Can you work these out from the model? Positions are in its coordinate system, mm. A direction names the side the tool comes from. Round coordinates to 2 decimals unless told otherwise and drop trailing zeros. Write each loop counter-clockwise with the first axis right and the second up, starting at its lowest first coordinate (ties: lowest second). Pieces come first, ordered by that corner, then holes. Notation, with made-up numbers: (-36.75, 55) - (-14.75, 55) arc R14 cw to (-14.75, 72) - close; hole circle Ø7 at (84.5, -7). An arc over 180 degrees is marked (long way). One line per item, written item: value. Start each with the question number.
(1) I want a section at A-A on z = 4.75. List the corners of the cut face in (x, y) for me, plus the area to 3 significant figures.
(2) On a 3-axis mill with a long thin cutter (end or side, diameter ignored), from which of +Z, -Z, +X, -X, +Y, -Y can I reach the whole of each face in a straight line? I mean faces 1 (the face through (4.7, 3, -11)), 2 (the face through (-6.6, 1.46, -2.8)), 3 (the face through (4.7, 4, 10)), 4 (the face through (-1, 3, -10)), 5 (the face through (-6.4, 3.2, -1.85)). Say none if no direction works.
(3) I want a section at C-C on z = -4.75. List the corners of the cut face in (x, y) for me.
(4) I want a section at B-B on x = 2.2. List the corners of the cut face in (y, z) for me.
(5) If I drill on L1, parallel to Z at x = 2.2, y = 4.25; L2, parallel to X at y = 1.75, z = 4.75; L3, parallel to X at y = 1.75, z = -4.75, over which ranges is the centre line in solid material (lowest first)? Write a range as from..to.
(6) I'm going to push flat-ended pins straight in: pin 1 Ø3 at (y, z) = (4.5, 2.5) entering from -X; pin 2 Ø1 at (x, y) = (-0.5, 1.5) entering from -Z; pin 3 Ø1.5 at (y, z) = (3, -11) entering from -X. Where does each tip first touch, or does it pass through?
(7) Thinking about a two-plate mould opening in Z: for faces 6 (the face through (4.928, 3.4, 9.667)), 7 (the face through (-5, 3, 5)), 8 (the face through (1.93, 3.22, -3.53)), 9 (the face through (0, 3, 10)), which applies, +Z half, -Z half, draft (parallel to the pull), parting line (faces both ways), or undercut?
(8) I want a section at D-D on x = -0.5. List the corners of the cut face in (y, z) for me, plus the area to 3 significant figures.
Autodesk Inventor part; units mm, degrees
ref_plane "YZ Plane" through (0, 0, 0) normal (1, 0, 0) x (0, 1, 0)
ref_plane "XZ Plane" through (0, 0, 0) normal (0, 1, 0) x (-1, 0, 0)
ref_plane "XY Plane" through (0, 0, 0) normal (0, 0, 1) x (1, 0, 0)
sketch "Skizze1" plane through (0, 0, 0) normal (0, 1, 0) x (-1, 0, 0)
  line L0 (5, 10) -> (-5, 10)
  line L1 (-5, 10) -> (-5, -10)
  line L2 (-5, -10) -> (5, -10)
  line L3 (5, -10) -> (5, 10)
  line L4 (5, 10) -> (-5, -10) construction
  line L5 (-5, 10) -> (5, -10) construction
  line L6 (5, -10) -> (6, -10)
  line L7 (6, -10) -> (6, 0)
  line L8 (6, 0) -> (5, 0)
  line L9 (5, 0) -> (5, -10)
  point P0 (0, 0)
  dimension "d0" = 10
  dimension "d1" = 20
  dimension "d2" = 1
extrude "Extrusion1" add sketch "Skizze1" along normal blind 6.35
sketch "Skizze2" plane through (-6, 0, -10) normal (-1, 0, 0) x (0, 0, 1)
  line L0 (0, 0) -> (0, 6.35)
  line L1 (0, 0) -> (10, 0)
  line L2 (0, 6.35) -> (8.15, 6.35)
  line L3 (8.15, 6.35) -> (8.15, 0)
  line L4 (8.15, 0) -> (0, 0)
  line L5 (0, 0) -> (0, 6.35)
  line L6 (8.15, 6.35) -> (6.15, 6.35)
  line L7 (6.15, 6.35) -> (6.15, 0)
  line L8 (6.15, 0) -> (8.15, 0)
  line L9 (8.15, 0) -> (8.15, 6.35)
  line L10 (6.15, 4.89) -> (8.15, 4.89)
  line L11 (8.15, 4.89) -> (8.15, 1.46)
  line L12 (8.15, 1.46) -> (6.15, 1.46)
  line L13 (6.15, 1.46) -> (6.15, 4.89)
  line L14 (6.15, 4.89) -> (8.15, 1.46) construction
  line L15 (8.15, 4.89) -> (6.15, 1.46) construction
  point P0 (7.15, 3.175)
  point P1 (8.15, 1.46)
  dimension "d5" = 8.15
  dimension "d6" = 2
  dimension "d7" = 2
  dimension "d8" = 3.43
extrude "Extrusion2" add sketch "Skizze2" along normal blind 1.15 contours L7 L10 L3 L12
sketch "Skizze3" plane through (-6, 4.89, -1.85) normal (0, 1, 0) x (1, 0, 0)
  line L0 (0, 2) -> (0, 0)
  line L1 (0, 2) -> (-1.15, 2)
  line L2 (-1.15, 0) -> (-1.15, 2)
  line L3 (0, 0) -> (-1.15, 0)
  circle A0 centre (1.35, 1) radius 2.5
  point P0 (6, -1.85)
  point P1 (-1.15, 1)
  point P2 (-0.9413, 0)
  point P3 (-0.9413, 2)
  dimension "d11" = 5
extrude "Extrusion3" cut sketch "Skizze3" against normal through all contours A0 L2 L1 | L3 L2 A0
fillet "Rundung1" radius 0.2 2 edges at (-6.9413, 3.175, -1.85) (-6.9413, 3.175, -3.85)
chamfer "Fase1" distance 1 angle 45 1 edges at (-6, 3.175, 0)
fillet "Rundung2" radius 0.2 4 edges at (-5, 3.175, 10) (5, 3.175, 10) (5, 3.175, -10) (-6, 3.175, -10)
move faces "Verschieben1" translate (-0.4, 0, 0) faces at (4.8149, 2.1167, 9.9994) (4.936, 2.1167, -9.9466) (5, 2.1167, 3.2667)
sketch "Skizze4" plane through (4.6, 0, 9.8) normal (1, 0, 0) x (0, 0, -1)
  line L0 (19.6, 6.35) -> (19.6, 0)
  line L1 (0, 6.35) -> (19.6, 6.35)
  line L2 (0, 0) -> (0, 6.35)
  line L3 (0, 0) -> (19.6, 0)
  line L4 (1.95, 4.725) -> (17.65, 4.725)
  line L5 (17.65, 4.725) -> (17.65, 1.625)
  line L6 (17.65, 1.625) -> (1.95, 1.625)
  line L7 (1.95, 1.625) -> (1.95, 4.725)
  line L8 (9.8, 0) -> (9.8, 6.35)
  line L9 (1.95, 4.725) -> (17.65, 1.625) construction
  line L10 (17.65, 4.725) -> (1.95, 1.625) construction
  line L11 (1.5, 4.725) -> (18.1, 4.725)
  line L12 (18.1, 4.725) -> (18.1, 1.625)
  line L13 (18.1, 1.625) -> (1.5, 1.625)
  line L14 (1.5, 1.625) -> (1.5, 4.725)
  line L15 (1.5, 4.725) -> (18.1, 1.625) construction
  line L16 (18.1, 4.725) -> (1.5, 1.625) construction
  line L17 (9.8, 4.725) -> (9.35, 4.725)
  line L18 (9.35, 4.725) -> (9.35, 1.625)
  line L19 (9.35, 1.625) -> (9.8, 1.625)
  line L20 (9.8, 1.625) -> (9.8, 4.725)
  point P0 (9.8, 3.175)
  point P1 (9.8, 3.175)
  point P2 (17.65, 4.725)
  point P3 (17.65, 1.625)
  point P4 (9.35, 4.725)
  point P5 (9.8, 1.625)
  point P6 (9.8, 4.725)
  point P7 (1.95, 1.625)
  point P8 (1.95, 4.725)
  dimension "d22" = 15.7
  dimension "d23" = 3.1
  dimension "d24" = 16.6
  dimension "d25" = 0.45
extrude "Extrusion4" add sketch "Skizze4" along normal blind 0.55 contours L8 L6 L18 L4 | L11 L12 L13 L5 | L7 L13 L14 L11
sketch "Skizze5" plane through (4.6, 4.725, 8.3) normal (0, 1, 0) x (1, 0, 0)
  line L0 (0, 0) -> (0, 0.45)
  line L1 (0, 0) -> (0.55, 0)
  line L2 (0.55, 0.45) -> (0.55, 0)
  line L3 (0, 0.45) -> (0.55, 0.45)
  line L4 (0, 16.15) -> (0, 16.6)
  line L5 (0, 16.15) -> (0.55, 16.15)
  line L6 (0.55, 16.6) -> (0.55, 16.15)
  line L7 (0, 16.6) -> (0.55, 16.6)
  line L8 (1, -4.015) -> (0.1, -4.015)
  line L9 (0.1, -4.015) -> (0.1, 20.615)
  line L10 (0.1, 20.615) -> (1, 20.615)
  line L11 (1, 20.615) -> (1, -4.015)
  line L12 (0.55, 7.85) -> (0.55, 8.3)
  line L13 (1, -4.015) -> (0.1, 20.615) construction
  line L14 (0.1, -4.015) -> (1, 20.615) construction
  line L15 (0.55, 20.615) -> (0.55, -4.015)
  point P0 (-4.6, 8.3)
  point P1 (0.1, 16.6)
  point P2 (0.1, 0)
  dimension "d28" = 0.9
  dimension "d29" = 24.63
extrude "Extrusion5" add sketch "Skizze5" against normal up to surface (3.1 mm away) contours L1 L15 L8 L9 | L9 L10 L15 L7
fillet "Rundung3" radius 0.2 2 edges at (5.15, 3.175, -7.85) (5.15, 3.175, 7.85)
fillet "Rundung4" radius 0.1 2 edges at (4.7, 3.175, -8.3) (4.7, 3.175, 8.3)
fillet "Rundung5" radius 0.1 2 edges at (5.15, 3.175, 0.45) (5.15, 3.175, 0)
sketch "Skizze6" plane through (5.15, 0, 9.8) normal (1, 0, 0) x (0, 0, -1)
  line L0 (1.75, 4.725) -> (1.75, 1.625)
  line L1 (1.75, 4.725) -> (-2.515, 4.725)
  line L2 (-2.515, 4.725) -> (-2.515, 1.625)
  line L3 (-2.515, 1.625) -> (1.75, 1.625)
  line L4 (17.85, 1.625) -> (17.85, 4.725)
  line L5 (17.85, 1.625) -> (22.115, 1.625)
  line L6 (22.115, 4.725) -> (22.115, 1.625)
  line L7 (17.85, 4.725) -> (22.115, 4.725)
  circle A0 centre (-0.5825, 3.175) radius 0.75
  circle A1 centre (19.7825, 3.175) radius 0.75
  point P0 (9.8, 0)
  dimension "d35" = 1.5
  dimension "d36" = 1.5
extrude "Extrusion6" cut sketch "Skizze6" against normal up to surface (0.45 mm away) contours A0 | A1
sketch "Skizze7" plane through (0, 6.35, 0) normal (0, 1, 0) x (1, 0, 0)
  line L0 (3.45, 6) -> (0.95, 6)
  line L1 (0.95, 6) -> (0.95, -6)
  line L2 (0.95, -6) -> (3.45, -6)
  line L3 (3.45, -6) -> (3.45, 6)
  line L4 (3.45, 6) -> (0.95, -6) construction
  line L5 (0.95, 6) -> (3.45, -6) construction
  line L6 (3.45, 3.5) -> (0.95, 3.5)
  line L7 (0.95, 3.5) -> (0.95, -3.5)
  line L8 (0.95, -3.5) -> (3.45, -3.5)
  line L9 (3.45, -3.5) -> (3.45, 3.5)
  line L10 (3.45, 3.5) -> (0.95, -3.5) construction
  line L11 (0.95, 3.5) -> (3.45, -3.5) construction
  circle A0 centre (2.2, 4.75) radius 1.25
  circle A1 centre (2.2, -4.75) radius 1.25
  arc A2 (4.95, 7.85) -> (5.15, 8.05) centre (4.95, 8.05) ccw
  line L12 (5.15, 8.05) -> (5.15, 12.315)
  line L13 (5.15, 12.315) -> (4.7, 12.315)
  line L14 (4.7, 12.315) -> (4.7, 8.4)
  arc A3 (4.6, 8.3) -> (4.7, 8.4) centre (4.6, 8.4) ccw
  line L15 (4.6, 7.85) -> (4.6, 8.3)
  line L16 (4.6, 7.85) -> (4.95, 7.85)
  arc A4 (5.15, -8.05) -> (4.95, -7.85) centre (4.95, -8.05) ccw
  line L17 (4.6, -7.85) -> (4.95, -7.85)
  line L18 (4.6, -8.3) -> (4.6, -7.85)
  arc A5 (4.7, -8.4) -> (4.6, -8.3) centre (4.6, -8.4) ccw
  line L19 (4.7, -8.4) -> (4.7, -12.315)
  line L20 (4.7, -12.315) -> (5.15, -12.315)
  line L21 (5.15, -8.05) -> (5.15, -12.315)
  point P0 (0, 0)
  point P1 (2.2, 0)
  point P2 (2.2, 0)
  point P3 (2.2, 3.5)
  point P4 (2.2, 6)
  point P5 (2.2, 0)
  dimension "d39" = 2.5
  dimension "d40" = 12
  dimension "d41" = 2.5
  dimension "d42" = 7
  dimension "d43" = 1.7
  dimension "d44" = 24.63
  dimension "d45" = 12.315
  dimension "d46" = 2.95
extrude "Extrusion7" cut sketch "Skizze7" against normal through all contours A0 | A1
fillet "Rundung6" radius 0.6 4 edges at (4.925, 4.725, 12.315) (4.925, 1.625, 12.315) (4.925, 4.725, -12.315) (4.925, 1.625, -12.315)
properties part number "Glicky_3D"
Established:
1. outline: (-5, 0) - (0.95, 0) - (0.95, 6.35) - (-5, 6.35) - close; (3.45, 0) - (4.6, 0) - (4.6, 6.35) - (3.45, 6.35) - close
1. area: 45.1 mm2
2. face 1: -Z, +Y, -Y
2. face 2: +Z, -Z, -X, -Y
2. face 3: +Z, +Y, -Y
2. face 4: -Z, -X, +Y, -Y
2. face 5: +Z, -X, +Y, -Y
3. outline: (-6, 0) - (0.95, 0) - (0.95, 6.35) - (-6, 6.35) - close; (3.45, 0) - (4.6, 0) - (4.6, 6.35) - (3.45, 6.35) - close
4. outline: (0, -10) - (6.35, -10) - (6.35, -6) - (0, -6) - close; (0, -3.5) - (6.35, -3.5) - (6.35, 3.5) - (0, 3.5) - close; (0, 6) - (6.35, 6) - (6.35, 10) - (0, 10) - close
5. L1: -10..-6, -3.5..3.5, 6..10
5. L2: -5..0.95, 3.45..4.6
5. L3: -6..0.95, 3.45..4.6
6. pin 1: x = -5
6. pin 2: z = -10
6. pin 3: x = 4.7
7. face 6: undercut
7. face 7: draft
7. face 8: undercut
7. face 9: +Z half
8. outline: (0, -10) - (6.35, -10) - (6.35, 10) - (0, 10) - close
8. area: 127 mm2
